```python
from build123d import *

# Parameters (mm, degrees)
F1_DEPTH = 63.5
F0_W     = 38.5974588745
F0_H     = 19.05
F2_DEPTH = 25.4
F3_DEPTH = 12.7


with BuildPart() as f1:
    # F0 (on Front) → F1 (new body, symmetric)
    with BuildSketch(Plane.XZ):
        Polygon((22.225, 9.525), (-41.275, 9.525), (-41.275, -9.525), (41.275, -9.525), (41.275, 9.525), align=None)
    extrude(amount=F1_DEPTH, both=True)

    # F0 (on Front) → F2 (join, symmetric)
    with BuildSketch(Plane.XZ):
        with BuildLine():
            Line((22.225, 27.2184735426), (22.225, 9.525))
            Line((22.225, 9.525), (41.275, 9.525))
            Line((41.275, 9.525), (41.275, 27.2184735426))
            ThreePointArc((41.275, 27.2184735426), (45.032594125, 37.4744035277), (54.5265401398, 42.8752))
            Line((54.5265401398, 42.8752), (60.325, 42.8752))
            Line((60.325, 42.8752), (60.325, 61.9252))
            Line((60.325, 61.9252), (53.2514408289, 61.9252))
            ThreePointArc((53.2514408289, 61.9252), (31.1124040659, 50.495054541), (22.225, 27.2184735426))
        make_face()
        with Locations((79.6237294372, 52.4002)):
            Rectangle(F0_W, F0_H)
    extrude(amount=F2_DEPTH, both=True)

    # F0 (on Front) → F3 (join, symmetric)
    with BuildSketch(Plane.XZ):
        with BuildLine():
            add(Edge.make_bspline(
                [(-41.275, 9.525), (-25.43013841, 42.0579750838), (17.2982045757, 61.6761899298), (53.2514408289, 61.9252)],
                knots=[0, 0, 0, 0, 108.0788090969, 108.0788090969, 108.0788090969, 108.0788090969], degree=3))
            Line((-41.275, 9.525), (22.225, 9.525))
            Line((22.225, 9.525), (22.225, 27.2184735426))
            ThreePointArc((22.225, 27.2184735426), (31.1124040659, 50.495054541), (53.2514408289, 61.9252))
        make_face()
    extrude(amount=F3_DEPTH, both=True)


solid = f1.part
```
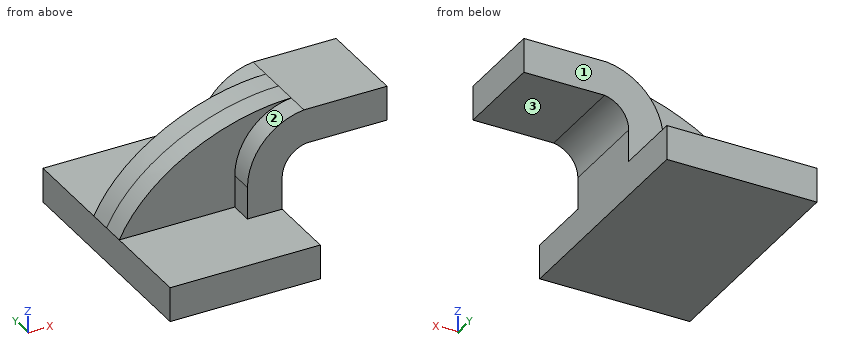
The listing builds one solid part. Answer for the finished solid, in the listing's coordinates (mm). Face numbers are marked on the shaded views. A direction names the side the tool comes from. Give positions to 0.01 mm unless a question says otherwise; leave off trailing zeros. Order: outer loops, then holes, each group sorted by start corner. A loop starts at its lowest first (then second) coordinate and runs counter-clockwise, first axis right, second up. Notation, with made-up numbers: M -36.75,80.25 L -15.75,80.25 A15 ccw -15.75,92.25 Z; hole C 54,22.5 d5. An arc over 180 degrees is marked long. Put each result on its own line as item: value. Start each with the question number.
Item 1: The part is cut by section C-C, the plane x = 75.5. Determine the outline of the cut face in (y, z), and give its area (3 significant figures).
Item 2: The part is cut by section A-A, the plane y = -22. Determine the outline of the cut face in (x, z) (3 decimals).
Item 3: Find the intervals of material crossed by line 1 along Z through (x, y) = (-11, 56.5) (3 decimals); line 2 along Y through (x, z) = (52.5, 52.5); line 3 along Z through (x, y) = (84, 22), in increasing order.
Item 4: The part is cut by section B-B, the plane z = -1.5. Determine the outline of the cut face in (x, y) (3 decimals), and give its area (3 significant figures).
Item 5: Flat-ended cylindrical pins translate along their axes: P1, Ø10, axis at x = 41, z = 17.5, coming from the -Y side; P2, Ø4, axis at y = 21, z = 16.5, coming from the -X side (3 decimals); P3, Ø1, axis at x = 41.5, z = 10.5, coming from the +Y side. Find the tip coordinate at first contact, or state that the pin passes through.
Item 6: Which of the six approach directions +Z, -Z, +X, -X, +Y, -Y give full straight-line access (tool end or side, diameter ignored) to the marked faces 1, 2 and 3?
Answer key:
1. outline: M -25.4,42.88 L 25.4,42.88 L 25.4,61.93 L -25.4,61.93 Z
1. area: 968 mm²
2. outline: M -41.275,-9.525 L 41.275,-9.525 L 41.275,27.218 A15.875 cw 54.527,42.875 L 98.922,42.875 L 98.922,61.925 L 53.251,61.925 A34.925 ccw 22.225,27.218 L 22.225,9.525 L -41.275,9.525 Z
3. line 1: z = -9.525 to 9.525
3. line 2: y = -25.4 to 25.4
3. line 3: z = 42.88 to 61.93
4. outline: M -41.275,-63.5 L 41.275,-63.5 L 41.275,63.5 L -41.275,63.5 Z
4. area: 10,500 mm²
5. P1: stops at y = -25.4
5. P2: stops at x = 22.225
5. P3: stops at y = 25.4
6. face 1: +Z, +X, -X, +Y
6. face 2: +Z, -X, -Y
6. face 3: -Z, +X, +Y, -Y
